from build123d import *

# Parameters (mm, degrees)
SKETCH1_R           = 1.984375
SKETCH1_R_2         = 1.190625
BOSS_EXTRUDE1_DEPTH = 61.9125
CHAMFER1_SIZE       = 0.254


with BuildPart() as part:
    # Sketch1 → Boss-Extrude1 (new body, symmetric)
    with BuildSketch(Plane(origin=(0, 0, 0), x_dir=(1, 0, 0), z_dir=(0, 1, 0))):
        Circle(SKETCH1_R)
        Circle(SKETCH1_R_2, mode=Mode.SUBTRACT)
    extrude(amount=BOSS_EXTRUDE1_DEPTH, both=True)

    # Chamfer1
    chamfer1_edges = [part.edges().sort_by_distance(p)[0] for p in [
        (-1.984375, -61.9125, 0),
        (-1.984375, 61.9125, 0),
        (-1.190625, -61.9125, 0),
        (-1.190625, 61.9125, 0),
    ]]
    chamfer(chamfer1_edges, length=CHAMFER1_SIZE)


solid = part.part
Check sheet for the modelled part. Datum: model origin and axes. Units: mm. Round coordinates to 2 decimals unless told otherwise and drop trailing zeros. Loops run counter-clockwise (first coordinate to the right, second up) from the corner with the lowest first, then second, coordinate; pieces in that order, holes last. Notation, with made-up numbers: M 34,74 L 75,74 A28 cw 75,94 Z; hole C -34,-27.75 d4. An arc over 180 degrees is marked long. One line per item, written item: value.
(1) Depth check by flat-ended pin: pin 1 Ø1 at (y, z) = (-23.5, 1) entering from +X; pin 2 Ø1.5 at (x, y) = (-1, 43.5) entering from -Z. Enter the tip coordinate at first touch or a pass-through.
Computed values:
pin 1: stops at x = 1.92
pin 2: stops at z = -1.97
(2) Sectioned sample at A-A, the plane z = 0. Record the cut outline in (x, y), then the cut area to 3 significant figures.
Computed values:
outline: M -1.98,-61.66 L -1.73,-61.91 L -1.44,-61.91 L -1.19,-61.66 L -1.19,61.66 L -1.44,61.91 L -1.73,61.91 L -1.98,61.66 Z; M 1.19,-61.66 L 1.44,-61.91 L 1.73,-61.91 L 1.98,-61.66 L 1.98,61.66 L 1.73,61.91 L 1.44,61.91 L 1.19,61.66 Z
area: 196 mm^2
(3) Sectioned sample at B-B, the plane x = 0. Record the cut outline in (y, z), then the cut area to 3 significant figures.
Computed values:
outline: M -61.91,-1.73 L -61.66,-1.98 L 61.66,-1.98 L 61.91,-1.73 L 61.91,-1.44 L 61.66,-1.19 L -61.66,-1.19 L -61.91,-1.44 Z; M -61.91,1.44 L -61.66,1.19 L 61.66,1.19 L 61.91,1.44 L 61.91,1.73 L 61.66,1.98 L -61.66,1.98 L -61.91,1.73 Z
area: 196 mm^2
(4) Release check for a two-part mould opening along Z. For faces 1 (the face through (-0.945, -0.863, 0.724)), 2 (the face through (-0.43, 0.863, 1.937)) record: +Z half, -Z half, draft (parallel to the pull), parting line (faces both ways), or undercut.
Computed values:
face 1: undercut
face 2: parting line
(5) Thickness scan on line 1 (Z direction, x = 0, y = 34); line 2 (Y direction, x = -1.25, z = 1.2). Record the ranges inside material, lowest first.
Computed values:
line 1: z = -1.98 to -1.19, 1.19 to 1.98
line 2: y = -61.91 to 61.91
(6) Sectioned sample at C-C, the plane y = 34. Record the cut outline in (x, z).
Computed values:
outline: C 0,0 d3.97; hole C 0,0 d2.38
